Check sheet for the modelled part. Datum: model origin and axes. Units: mm. A direction names the side the tool comes from. Round coordinates to 2 decimals unless told otherwise and drop trailing zeros. Order: outer loops, then holes, each group sorted by start corner. A loop starts at its lowest first (then second) coordinate and runs counter-clockwise, first axis right, second up. Notation, with made-up numbers: (-39.75, 7) -> (-16.75, 7) arc R24 cw to (-16.75, 28) -> close; hole circle Ø3 at (75, 59.25). An arc over 180 degrees is marked (long way). Answer in a Markdown table with one row per item. Add a question column.
1. Access from +Z, -Z, +X, -X, +Y, -Y to the whole of each face (thin tool, end or side, straight path). Record for faces 4 (the cylindrical face through (-18.54, 0.43, -31.83)), 5 (the flat face through (-10, -5, 5)), 6 (the flat face through (-29.232, 4.104, 16.731)).
2. Draft check along X on faces 1 (the flat face through (30.834, 4.104, 17.957)), 2 (the cylindrical face through (18.549, 0.451, 31.848)), 3 (the cylindrical face through (-18.29, 0.43, 31.97)). Enter one of: +X half, -X half, draft (parallel to the pull), parting line (faces both ways), or undercut.
3. Depth check by flat-ended pin: P1, Ø0.7, axis at x = 4, y = 4, coming from the -Z side; P2, Ø4, axis at y = -5.5, z = -4.5, coming from the +X side; P3, Ø5, axis at y = -1, z = 19, coming from the +X side. Enter the tip coordinate at first touch or a pass-through.
4. Sectioned sample at A-A, the plane y = -5. Record the boundary of the cut face in (x, z), then the cut area to 3 significant figures.
5. Sectioned sample at B-B, the plane x = -5. Count the separate pieces of the cut face and the enclosed holes in it, then the cut area to 3 significant figures.
6. Material ranges on L1, parallel to X at y = -5, z = -4.5; L2, parallel to Y at x = 5, z = 4.75; L3, parallel to Z at x = 0, y = -2, recorded low to high. Write a range as from..to.
```python
from build123d import *

# Parameters (mm, degrees)
EXTRUDE_1_DEPTH          = 4.4
CUT_EXTRUDE_1_DEPTH      = 0.6
FILLET_1_R               = 1.5
SKETCH_3_W               = 20
SKETCH_3_H               = 15
EXTRUDE_2_DEPTH          = 10
SKETCH_4_W               = 20
SKETCH_4_H               = 5.2
CUT_EXTRUDE_2_DEPTH      = 10
CUT_EXTRUDE_3_DEPTH      = 60.123345338
CUT_EXTRUDE_3_DEPTH_BACK = 60.123345338
SKETCH_5_R               = 1.6


with BuildPart() as part:
    # 스케치1 → 보스-돌출1 (new body)
    with BuildSketch(Plane(origin=(0, 0, 0), x_dir=(1, 0, 0), z_dir=(0, 1, 0))):
        Polygon((27.293187568, -27.293187568), (37.283187568, -9.99), (37.283187568, 9.99), (27.293187568, 27.293187568), (9.99, 37.283187568), (-9.99, 37.283187568), (-27.293187568, 27.293187568), (-37.283187568, 9.99), (-37.283187568, -9.99), (-27.293187568, -27.293187568), (-9.99, -37.283187568), (9.99, -37.283187568), align=None)
    extrude(amount=EXTRUDE_1_DEPTH)

    # 스케치2 → 컷-돌출1 (cut)
    with BuildSketch(Plane(origin=(0, 4.4, 0), x_dir=(1, 0, 0), z_dir=(0, 1, 0))):
        Polygon((-26.120860153, 26.120860153), (-35.681758538, 9.560898385), (-35.681758538, -9.560898385), (-26.120860153, -26.120860153), (-9.560898385, -35.681758538), (9.560898385, -35.681758538), (26.120860153, -26.120860153), (35.681758538, -9.560898385), (35.681758538, 9.560898385), (26.120860153, 26.120860153), (9.560898385, 35.681758538), (-9.560898385, 35.681758538), align=None)
        Polygon((24.656758538, -24.656758538), (33.681758538, -9.025), (33.681758538, 9.025), (24.656758538, 24.656758538), (9.025, 33.681758538), (-9.025, 33.681758538), (-24.656758538, 24.656758538), (-33.681758538, 9.025), (-33.681758538, -9.025), (-24.656758538, -24.656758538), (-9.025, -33.681758538), (9.025, -33.681758538), align=None, mode=Mode.SUBTRACT)
    extrude(amount=-CUT_EXTRUDE_1_DEPTH, mode=Mode.SUBTRACT)

    # 필렛1
    fillet_1_edges = [part.edges().sort_by_distance(p)[0] for p in [
        (0, 0, 37.283187568),
        (-18.641593784, 0, 32.288187568),
        (37.283187568, 4.4, 0),
        (-32.288187568, 0, 18.641593784),
        (-37.283187568, 0, 0),
        (-32.288187568, 0, -18.641593784),
        (-18.641593784, 0, -32.288187568),
        (0, 0, -37.283187568),
        (18.641593784, 0, -32.288187568),
        (32.288187568, 0, -18.641593784),
        (37.283187568, 0, 0),
        (32.288187568, 0, 18.641593784),
        (18.641593784, 0, 32.288187568),
        (32.288187568, 4.4, -18.641593784),
        (18.641593784, 4.4, -32.288187568),
        (0, 4.4, -37.283187568),
        (-18.641593784, 4.4, -32.288187568),
        (-32.288187568, 4.4, -18.641593784),
        (-37.283187568, 4.4, 0),
        (-32.288187568, 4.4, 18.641593784),
        (-18.641593784, 4.4, 32.288187568),
        (0, 4.4, 37.283187568),
        (18.641593784, 4.4, 32.288187568),
        (32.288187568, 4.4, 18.641593784),
    ]]
    fillet(fillet_1_edges, radius=FILLET_1_R)

    # 스케치3 → 보스-돌출2 (add)
    with BuildSketch(Plane.XZ):
        Rectangle(SKETCH_3_W, SKETCH_3_H)
    extrude(amount=EXTRUDE_2_DEPTH)

    # 스케치4 → 컷-돌출2 (cut)
    with BuildSketch(Plane.XZ.offset(10)):
        Rectangle(SKETCH_4_W, SKETCH_4_H)
    extrude(amount=-CUT_EXTRUDE_2_DEPTH, mode=Mode.SUBTRACT)

    # 스케치5 → 컷-돌출3 (cut, two sides: drawn at the far end of the back side and taken through both)
    with BuildSketch(Plane(origin=(0, 0, -7.5), x_dir=(-1, 0, 0), z_dir=(0, 0, -1)).offset(-CUT_EXTRUDE_3_DEPTH_BACK)):
        with Locations((-5, -5)):
            Circle(SKETCH_5_R)
        with Locations((5, -5)):
            Circle(SKETCH_5_R)
    extrude(amount=CUT_EXTRUDE_3_DEPTH + CUT_EXTRUDE_3_DEPTH_BACK, mode=Mode.SUBTRACT)


solid = part.part
```
Answer key:
| question | item | result |
|---|---|---|
| 1 | face 4 | -Z, -X, -Y |
| 1 | face 5 | +Z, -Z, -X, -Y |
| 1 | face 6 | +Y |
| 2 | face 1 | undercut |
| 2 | face 2 | +X half |
| 2 | face 3 | -X half |
| 3 | P1 | stops at z = -37.08 |
| 3 | P2 | stops at x = 10 |
| 3 | P3 | stops at x = 32.88 |
| 4 | outline | (-10, -7.5) -> (-6.6, -7.5) -> (-6.6, -2.6) -> (-10, -2.6) -> close; (-10, 2.6) -> (-6.6, 2.6) -> (-6.6, 7.5) -> (-10, 7.5) -> close; (-3.4, -7.5) -> (3.4, -7.5) -> (3.4, -2.6) -> (-3.4, -2.6) -> close; (-3.4, 2.6) -> (3.4, 2.6) -> (3.4, 7.5) -> (-3.4, 7.5) -> close; (6.6, -7.5) -> (10, -7.5) -> (10, -2.6) -> (6.6, -2.6) -> close; (6.6, 2.6) -> (10, 2.6) -> (10, 7.5) -> (6.6, 7.5) -> close |
| 4 | area | 133 mm² |
| 5 | separate pieces | 3 |
| 5 | enclosed holes | 0 |
| 5 | area | 390 mm² |
| 6 | L1 | x = -10..-6.6, -3.4..3.4, 6.6..10 |
| 6 | L2 | y = -10..-6.6, -3.4..4.4 |
| 6 | L3 | z = -7.5..-2.6, 2.6..7.5 |
